from build123d import *

# Parameters (mm, degrees)
SKETCH_1_R      = 19.783013461
EXTRUDE_1_DEPTH = 130
EXTRUDE_2_DEPTH = 80


with BuildPart() as part:
    # 草图1 → 凸台-拉伸1 (new body)
    with BuildSketch(Plane.XY):
        Circle(SKETCH_1_R)
    extrude(amount=EXTRUDE_1_DEPTH)

    # 草图2 → 凸台-拉伸2 (add)
    with BuildSketch(Plane(origin=(0, 0, 0), x_dir=(-1, 0, 0), z_dir=(0, 0, -1))):
        with BuildLine():
            Line((-20.351449461, 40.092355437), (-20.351449461, 15.61573037))
            Line((-20.351449461, 15.61573037), (-42.163105017, 15.61573037))
            ThreePointArc((-42.163105017, 15.61573037), (-44.961966813, 0), (-42.163105017, -15.61573037))
            Line((-42.163105017, -15.61573037), (-20.351449461, -15.61573037))
            Line((-20.351449461, -15.61573037), (-20.351449461, -40.092355437))
            ThreePointArc((-20.351449461, -40.092355437), (0.671443732, -44.956952999), (21.539684559, -39.466700505))
            Line((21.539684559, -39.466700505), (21.183464145, -15.61573037))
            Line((21.183464145, -15.61573037), (42.163105017, -15.61573037))
            ThreePointArc((42.163105017, -15.61573037), (44.961966813, 0), (42.163105017, 15.61573037))
            Line((42.163105017, 15.61573037), (20.717014193, 15.61573037))
            Line((20.717014193, 15.61573037), (20.351449461, 40.092355437))
            ThreePointArc((20.351449461, 40.092355437), (0, 44.961966813), (-20.351449461, 40.092355437))
        make_face()
    extrude(amount=EXTRUDE_2_DEPTH)

    # 草图4 → 放样1 section 0
    with BuildSketch(Plane(origin=(0, 0, -80), x_dir=(-1, 0, 0), z_dir=(0, 0, -1)), mode=Mode.PRIVATE) as loft_1_s0:
        with BuildLine():
            Line((-20.351449461, 15.61573037), (-42.163105017, 15.61573037))
            ThreePointArc((-42.163105017, 15.61573037), (-44.961966813, 0), (-42.163105017, -15.61573037))
            Line((-42.163105017, -15.61573037), (-20.351449461, -15.61573037))
            Line((-20.351449461, -15.61573037), (-20.351449461, -40.092355437))
            ThreePointArc((-20.351449461, -40.092355437), (0.671443732, -44.956952999), (21.539684559, -39.466700505))
            Line((21.539684559, -39.466700505), (21.183464145, -15.61573037))
            Line((21.183464145, -15.61573037), (42.163105017, -15.61573037))
            ThreePointArc((42.163105017, -15.61573037), (44.961966813, 0), (42.163105017, 15.61573037))
            Line((42.163105017, 15.61573037), (20.717014193, 15.61573037))
            Line((20.717014193, 15.61573037), (20.351449461, 40.092355437))
            ThreePointArc((20.351449461, 40.092355437), (0, 44.961966813), (-20.351449461, 40.092355437))
            Line((-20.351449461, 40.092355437), (-20.351449461, 15.61573037))
        make_face()
    loft([loft_1_s0.sketch, Vertex(0, 0, -100)])


solid = part.part
Geometry: final body of the model. Coordinates: model frame, mm. A direction names the side the tool comes from. Coordinates: 2 decimals unless noted, no trailing zeros. Order: outer loops, then holes, each group sorted by start corner. A loop starts at its lowest first (then second) coordinate and runs counter-clockwise, first axis right, second up.
1) Section B-B (z = 27.5). Return loops of the section in (x, y).
Result sheet:
outline: circle Ø39.57 at (0, 0)
2) Set-up query: faces 1 (the flat face through (20.351, 28, -39)), 2 (the flat face through (21.18, -10.085, -87.084)), 3 (the flat face through (20.983, 10.663, -86.343)), 4 (the flat face through (31, -15.616, -39)), 5 (the flat face through (-21.18, 10.663, -86.343)). Return all of +Z, -Z, +X, -X, +Y, -Y with unobstructed straight access to the full face (end or side cutting, diameter ignored); none if empty.
Result sheet:
face 1: +Z, -Z, +X, +Y
face 2: -Z, +X, -Y
face 3: -Z, +X, +Y
face 4: +Z, -Z, +X, -Y
face 5: -Z, -X, +Y
3) Ray query, probe 1 along Y at (x, z) = (34.5, -28); probe 2 along X at (y, z) = (-16, -45); probe 3 along Z at (x, y) = (-7, -39). Return the intervals inside material, ascending.
Result sheet:
probe 1: y = -15.62 to 15.62
probe 2: x = -21.19 to 20.35
probe 3: z = -82.37 to 0
4) First-contact query: P1, Ø1.5, axis at x = 34, y = -14, coming from the +Z side; P2, Ø3, axis at x = 11, y = -3.5, coming from the -Z side; P3, Ø6.5, axis at x = -31, z = -22, coming from the -Y side; P4, Ø2, axis at x = -22, z = 52.5, coming from the -Y side. Flat tips, straight axial feed; report the tip coordinate or a pass-through.
Result sheet:
P1: stops at z = 0
P2: stops at z = -95.53
P3: stops at y = -15.62
P4: passes through
5) Section A-A (z = -43). Return loops of the section in (x, y), then the cut area to 3 significant figures.
Result sheet:
outline: (-42.16, -15.62) - (-21.18, -15.62) - (-21.54, -39.47) arc R44.96 ccw to (20.35, -40.09) - (20.35, -15.62) - (42.16, -15.62) arc R44.96 ccw to (42.16, 15.62) - (20.35, 15.62) - (20.35, 40.09) arc R44.96 ccw to (-20.35, 40.09) - (-20.72, 15.62) - (-42.16, 15.62) arc R44.96 ccw to start
area: 5,040 mm2
